Study the drawing (mm; zero at the part's minimum x, y, z) and answer. Round coordinates to 2 decimals unless told otherwise and drop trailing zeros. Order: outer loops, then holes, each group sorted by start corner. A loop starts at its lowest first (then second) coordinate and runs counter-clockwise, first axis right, second up. Notation, with made-up numbers: (-11, 60.5) - (45, 60.5) arc R24 cw to (45, 70.5) - close; hole circle Ø3 at (71.25, 0). An arc over 180 degrees is marked (long way). Put each result on its own line as item: value. Start each with the question number.
Q1. For a pull along Y with two mould halves and no side action, classify the marked faces 1, 2, 3 and 4 as pulls with the +Y half, pulls with the -Y half, needs draft (parallel to the pull), parting line crosses it, or undercut.
Q2. Section D-D on z = 12.25 is taken. Give the vertices of the cut face in (x, y).
Q3. Section C-C on z = 4 is taken. Give the vertices of the cut face in (x, y), then the cut area to 3 significant figures.
Q4. Each of these flat-tipped pins is pushed along its axis until it touches: pin 1 Ø1 at (x, z) = (4.5, 7) entering from -Y; pin 2 Ø7 at (x, y) = (9, 9) entering from +Z; pin 3 Ø10 at (y, z) = (2.5, 17) entering from -X. Where does it stop, or does it pass through?
Q5. Find the intervals of material crossed by line 1 along Y through (x, z) = (9, 4); line 2 along Z through (x, y) = (11.25, 9.75); line 3 along Y through (x, z) = (9, 23.6), in increasing order. Write a range as from..to.
Q6. Section A-A on x = 9 is taken. Give the vertices of the cut face in (y, z).
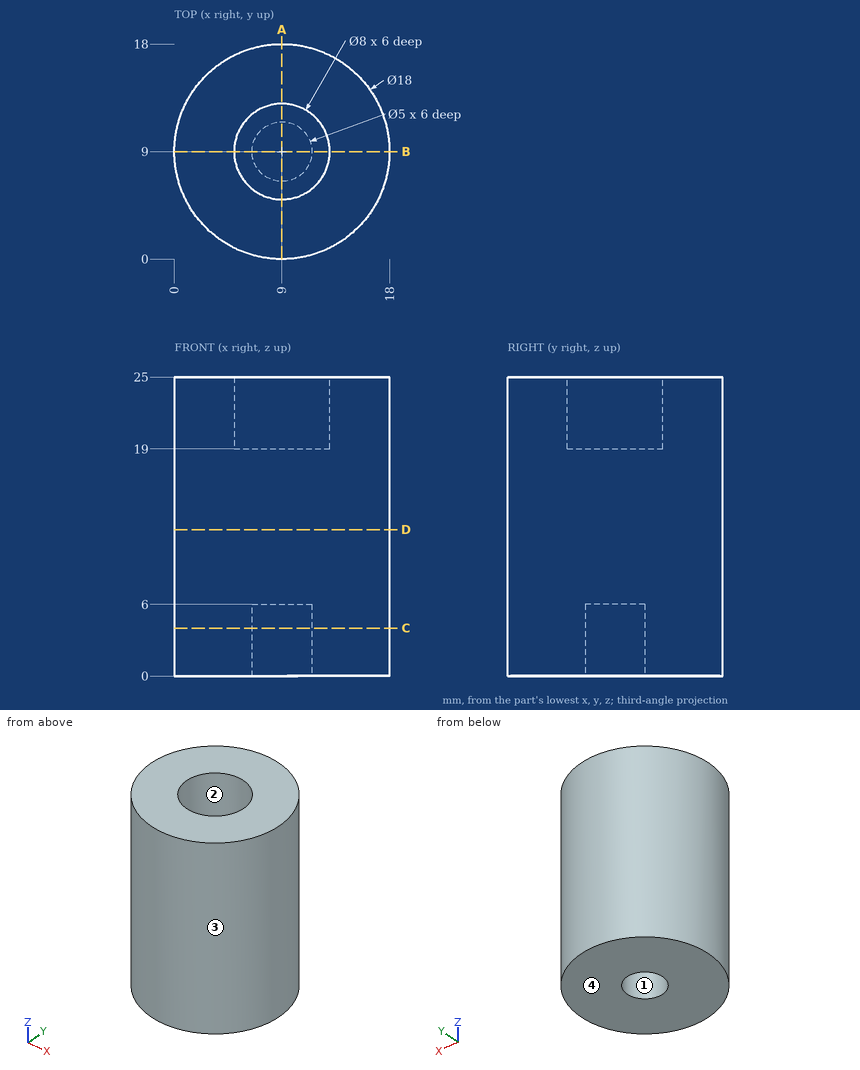
Findings:
1. face 1: undercut
1. face 2: undercut
1. face 3: parting line crosses it
1. face 4: needs draft
2. outline: circle Ø18 at (9, 9)
3. outline: circle Ø18 at (9, 9); hole circle Ø5 at (9, 9)
3. area: 235 mm2
4. pin 1: y = 0.94
4. pin 2: z = 19
4. pin 3: x = 0.13
5. line 1: 0..6.5, 11.5..18
5. line 2: 6..19
5. line 3: 0..5, 13..18
6. outline: (0, 0) - (6.5, 0) - (6.5, 6) - (11.5, 6) - (11.5, 0) - (18, 0) - (18, 25) - (13, 25) - (13, 19) - (5, 19) - (5, 25) - (0, 25) - close
